Could you check a few things on this model? Use its own coordinates, in mm. Face numbers are marked on the shaded views. Coordinates: 2 decimals unless noted, no trailing zeros. Write each loop counter-clockwise with the first axis right and the second up, starting at its lowest first coordinate (ties: lowest second). Pieces come first, ordered by that corner, then holes. Notation, with made-up numbers: (-35, 15.25) - (0, 15.25) arc R35 ccw to (0, 48.25) - close; hole circle Ø5 at (-24, -6). An arc over 180 degrees is marked (long way). Answer as a JSON object with one key per item and string values. Group by question number.
1) If we section it at D-D (x = 10): Write out the boundary of the cut face in (y, z), plus the area to 3 significant figures.
2) If we section it at B-B (x = -1.5): Write out the boundary of the cut face in (y, z).
3) Will these pins go through, and if not, where does the flat tip stop? pin 1 Ø0.5 at (y, z) = (0.5, 3) entering from +X; pin 2 Ø0.5 at (y, z) = (0.5, 0) entering from -X.
4) We'd pull the mould along Y, two halves only. Please class the marked faces 1 and 2: released by +Y, released by -Y, zero draft, split by the parting line, or undercut.
5) Please list where these lines run through material, in increasing order: line 1 along X through (y, z) = (0.5, 0); line 2 along Z through (x, y) = (3.5, 0.3); line 3 along Z through (x, y) = (11, 0.95).
6) If we section it at C-C (z = 14.5): Write out the boundary of the cut face in (x, y), plus the area to 3 significant figures.
```python
from build123d import *

# Parameters (mm, degrees)
SKETCH_3_R          = 35
EXTRUDE_1_DEPTH     = 2
SKETCH_4_W          = 5
SKETCH_4_H          = 0.8
CUT_EXTRUDE_6_DEPTH = 3
SKETCH_5_R          = 2.4
CUT_EXTRUDE_7_DEPTH = 3
CUT_EXTRUDE_8_DEPTH = 1


with BuildPart() as part:
    # 스케치3 → 보스-돌출1 (new body)
    with BuildSketch(Plane(origin=(0, 0, 0), x_dir=(1, 0, 0), z_dir=(0, 1, 0))):
        Circle(SKETCH_3_R)
    extrude(amount=EXTRUDE_1_DEPTH)

    # 스케치4 → 컷-돌출6 (cut, through all)
    with BuildSketch(Plane(origin=(0, 2, 0), x_dir=(1, 0, 0), z_dir=(0, 1, 0))):
        with Locations((-35, 0)):
            Rectangle(SKETCH_4_W, SKETCH_4_H)
        with Locations((35, 0)):
            Rectangle(SKETCH_4_W, SKETCH_4_H)
    extrude(amount=-CUT_EXTRUDE_6_DEPTH, mode=Mode.SUBTRACT)

    # 스케치5 → 컷-돌출7 (cut, through all)
    with BuildSketch(Plane(origin=(0, 2, 0), x_dir=(1, 0, 0), z_dir=(0, 1, 0))):
        Circle(SKETCH_5_R)
    extrude(amount=-CUT_EXTRUDE_7_DEPTH, mode=Mode.SUBTRACT)

    # 스케치6 → 컷-돌출8 (cut)
    with BuildSketch(Plane.XZ):
        Polygon((-22.083647797, 12.75), (-22.083647797, -12.75), (0, -25.5), (22.083647797, -12.75), (22.083647797, 12.75), (0, 25.5), align=None)
        Polygon((-20.883647797, 12.057179677), (-20.883647797, -12.057179677), (0, -24.114359354), (20.883647797, -12.057179677), (20.883647797, 12.057179677), (0, 24.114359354), align=None, mode=Mode.SUBTRACT)
    extrude(amount=-CUT_EXTRUDE_8_DEPTH, mode=Mode.SUBTRACT)


solid = part.part
```
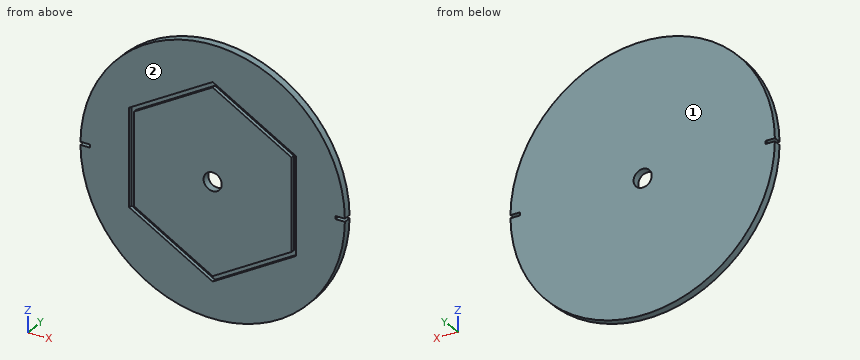
Here are the results:
{
 "1": {"outline": "(0, -33.54) - (2, -33.54) - (2, 33.54) - (0, 33.54) - (0, 19.73) - (1, 19.73) - (1, 18.34) - (0, 18.34) - (0, -18.34) - (1, -18.34) - (1, -19.73) - (0, -19.73) - close", "area": "131 mm²"},
 "2": {"outline": "(0, -34.97) - (2, -34.97) - (2, -1.87) - (0, -1.87) - (0, -23.25) - (1, -23.25) - (1, -24.63) - (0, -24.63) - close; (0, 1.87) - (2, 1.87) - (2, 34.97) - (0, 34.97) - (0, 24.63) - (1, 24.63) - (1, 23.25) - (0, 23.25) - close"},
 "3": {"pin 1": "stops at x = 34.89", "pin 2": "stops at x = -32.5"},
 "4": {"face 1": "released by +Y", "face 2": "released by -Y"},
 "5": {"line 1": "x = -32.5 to -22.08, -20.88 to -2.4, 2.4 to 20.88, 22.08 to 32.5", "line 2": "z = -34.82 to -23.48, -22.09 to 22.09, 23.48 to 34.82", "line 3": "z = -33.23 to -19.15, -17.76 to 17.76, 19.15 to 33.23"},
 "6": {"outline": "(-31.86, 0) - (-19.05, 0) - (-19.05, 1) - (-16.65, 1) - (-16.65, 0) - (16.65, 0) - (16.65, 1) - (19.05, 1) - (19.05, 0) - (31.86, 0) - (31.86, 2) - (-31.86, 2) - close", "area": "123 mm²"}
}
